Autodesk Inventor part; units mm, degrees
ref_plane "YZ Plane" through (0, 0, 0) normal (1, 0, 0) x (0, 1, 0)
ref_plane "XZ Plane" through (0, 0, 0) normal (0, 1, 0) x (-1, 0, 0)
ref_plane "XY Plane" through (0, 0, 0) normal (0, 0, 1) x (1, 0, 0)
sketch "Sketch1" plane through (0, 0, 0) normal (0, 0, 1) x (1, 0, 0)
  circle A0 centre (0, 0) radius 20.05
  dimension "d0" = 40.1
extrude "Extrusion1" add sketch "Sketch1" along normal blind 17.5
sketch "Sketch2" plane through (0, 0, 17.5) normal (0, 0, 1) x (1, 0, 0)
  line L0 (-16.51, 0) -> (-20.1782, -2.1178)
  line L1 (-20.1782, -2.1178) -> (-20.1782, 2.1178)
  line L2 (-20.1782, 2.1178) -> (-16.51, 0)
  line L3 (-16.1492, -3.4326) -> (-19.297, -6.2669)
  line L4 (-19.297, -6.2669) -> (-20.1776, -2.1237)
  line L5 (-20.1776, -2.1237) -> (-16.1492, -3.4326)
  line L6 (-15.0827, -6.7152) -> (-17.5723, -10.142)
  line L7 (-17.5723, -10.142) -> (-19.2951, -6.2725)
  line L8 (-19.2951, -6.2725) -> (-15.0827, -6.7152)
  line L9 (-13.3569, -9.7043) -> (-15.0797, -13.5738)
  line L10 (-15.0797, -13.5738) -> (-17.5694, -10.1471)
  line L11 (-17.5694, -10.1471) -> (-13.3569, -9.7043)
  line L12 (-11.0474, -12.2693) -> (-11.928, -16.4125)
  line L13 (-11.928, -16.4125) -> (-15.0757, -13.5782)
  line L14 (-15.0757, -13.5782) -> (-11.0474, -12.2693)
  line L15 (-8.255, -14.2981) -> (-8.255, -18.5338)
  line L16 (-8.255, -18.5338) -> (-11.9232, -16.4159)
  line L17 (-11.9232, -16.4159) -> (-8.255, -14.2981)
  line L18 (-5.1019, -15.702) -> (-4.2212, -19.8451)
  line L19 (-4.2212, -19.8451) -> (-8.2496, -18.5362)
  line L20 (-8.2496, -18.5362) -> (-5.1019, -15.702)
  line L21 (-1.7258, -16.4196) -> (-0.003, -20.2891)
  line L22 (-0.003, -20.2891) -> (-4.2154, -19.8463)
  line L23 (-4.2154, -19.8463) -> (-1.7258, -16.4196)
  line L24 (1.7258, -16.4196) -> (4.2154, -19.8463)
  line L25 (4.2154, -19.8463) -> (0.003, -20.2891)
  line L26 (0.003, -20.2891) -> (1.7258, -16.4196)
  line L27 (5.1019, -15.702) -> (8.2496, -18.5362)
  line L28 (8.2496, -18.5362) -> (4.2212, -19.8451)
  line L29 (4.2212, -19.8451) -> (5.1019, -15.702)
  line L30 (8.255, -14.2981) -> (11.9232, -16.4159)
  line L31 (11.9232, -16.4159) -> (8.255, -18.5338)
  line L32 (8.255, -18.5338) -> (8.255, -14.2981)
  line L33 (11.0474, -12.2693) -> (15.0757, -13.5782)
  line L34 (15.0757, -13.5782) -> (11.928, -16.4125)
  line L35 (11.928, -16.4125) -> (11.0474, -12.2693)
  line L36 (13.3569, -9.7043) -> (17.5694, -10.1471)
  line L37 (17.5694, -10.1471) -> (15.0797, -13.5738)
  line L38 (15.0797, -13.5738) -> (13.3569, -9.7043)
  line L39 (15.0827, -6.7152) -> (19.2951, -6.2725)
  line L40 (19.2951, -6.2725) -> (17.5723, -10.142)
  line L41 (17.5723, -10.142) -> (15.0827, -6.7152)
  line L42 (16.1492, -3.4326) -> (20.1776, -2.1237)
  line L43 (20.1776, -2.1237) -> (19.297, -6.2669)
  line L44 (19.297, -6.2669) -> (16.1492, -3.4326)
  line L45 (16.51, 0) -> (20.1782, 2.1178)
  line L46 (20.1782, 2.1178) -> (20.1782, -2.1178)
  line L47 (20.1782, -2.1178) -> (16.51, 0)
  line L48 (16.1492, 3.4326) -> (19.297, 6.2669)
  line L49 (19.297, 6.2669) -> (20.1776, 2.1237)
  line L50 (20.1776, 2.1237) -> (16.1492, 3.4326)
  line L51 (15.0827, 6.7152) -> (17.5723, 10.142)
  line L52 (17.5723, 10.142) -> (19.2951, 6.2725)
  line L53 (19.2951, 6.2725) -> (15.0827, 6.7152)
  line L54 (13.3569, 9.7043) -> (15.0797, 13.5738)
  line L55 (15.0797, 13.5738) -> (17.5694, 10.1471)
  line L56 (17.5694, 10.1471) -> (13.3569, 9.7043)
  line L57 (11.0474, 12.2693) -> (11.928, 16.4125)
  line L58 (11.928, 16.4125) -> (15.0757, 13.5782)
  line L59 (15.0757, 13.5782) -> (11.0474, 12.2693)
  line L60 (8.255, 14.2981) -> (8.255, 18.5338)
  line L61 (8.255, 18.5338) -> (11.9232, 16.4159)
  line L62 (11.9232, 16.4159) -> (8.255, 14.2981)
  line L63 (5.1019, 15.702) -> (4.2212, 19.8451)
  line L64 (4.2212, 19.8451) -> (8.2496, 18.5362)
  line L65 (8.2496, 18.5362) -> (5.1019, 15.702)
  line L66 (1.7258, 16.4196) -> (0.003, 20.2891)
  line L67 (0.003, 20.2891) -> (4.2154, 19.8463)
  line L68 (4.2154, 19.8463) -> (1.7258, 16.4196)
  line L69 (-1.7258, 16.4196) -> (-4.2154, 19.8463)
  line L70 (-4.2154, 19.8463) -> (-0.003, 20.2891)
  line L71 (-0.003, 20.2891) -> (-1.7258, 16.4196)
  line L72 (-5.1019, 15.702) -> (-8.2496, 18.5362)
  line L73 (-8.2496, 18.5362) -> (-4.2212, 19.8451)
  line L74 (-4.2212, 19.8451) -> (-5.1019, 15.702)
  line L75 (-8.255, 14.2981) -> (-11.9232, 16.4159)
  line L76 (-11.9232, 16.4159) -> (-8.255, 18.5338)
  line L77 (-8.255, 18.5338) -> (-8.255, 14.2981)
  line L78 (-11.0474, 12.2693) -> (-15.0757, 13.5782)
  line L79 (-15.0757, 13.5782) -> (-11.928, 16.4125)
  line L80 (-11.928, 16.4125) -> (-11.0474, 12.2693)
  line L81 (-13.3569, 9.7043) -> (-17.5694, 10.1471)
  line L82 (-17.5694, 10.1471) -> (-15.0797, 13.5738)
  line L83 (-15.0797, 13.5738) -> (-13.3569, 9.7043)
  line L84 (-15.0827, 6.7152) -> (-19.2951, 6.2725)
  line L85 (-19.2951, 6.2725) -> (-17.5723, 10.142)
  line L86 (-17.5723, 10.142) -> (-15.0827, 6.7152)
  line L87 (-16.1492, 3.4326) -> (-20.1776, 2.1237)
  line L88 (-20.1776, 2.1237) -> (-19.297, 6.2669)
  line L89 (-19.297, 6.2669) -> (-16.1492, 3.4326)
  point P0 (0, 0)
  point P1 (-18.9555, 0)
  point P2 (-18.5413, -3.9411)
  point P3 (-17.3167, -7.7099)
  point P4 (-15.3353, -11.1418)
  point P5 (-12.6837, -14.0867)
  point P6 (-9.4777, -16.4159)
  point P7 (-5.8576, -18.0277)
  point P8 (-1.9814, -18.8517)
  point P9 (1.9814, -18.8517)
  point P10 (5.8576, -18.0277)
  point P11 (9.4777, -16.4159)
  point P12 (12.6837, -14.0867)
  point P13 (15.3353, -11.1418)
  point P14 (17.3167, -7.7099)
  point P15 (18.5413, -3.9411)
  point P16 (18.9555, 0)
  point P17 (18.5413, 3.9411)
  point P18 (17.3167, 7.7099)
  point P19 (15.3353, 11.1418)
  point P20 (12.6837, 14.0867)
  point P21 (9.4777, 16.4159)
  point P22 (5.8576, 18.0277)
  point P23 (1.9814, 18.8517)
  point P24 (-1.9814, 18.8517)
  point P25 (-5.8576, 18.0277)
  point P26 (-9.4777, 16.4159)
  point P27 (-12.6837, 14.0867)
  point P28 (-15.3353, 11.1418)
  point P29 (-17.3167, 7.7099)
  point P30 (-18.5413, 3.9411)
  dimension "d5" = 360
extrude "Extrusion2" cut sketch "Sketch2" against normal through all
sketch "Sketch3" plane through (0, 0, 0) normal (0, 0, -1) x (-1, 0, 0)
  point P0 (0, 0)
  point P1 (0, 0)
hole "Hole1" at (0, 0, 0) at (0, 0, 0) direction (0, 0, 1) diameter 6 end through all
properties part number "gear(1.5 inch with 2mm extra)"
Could you check a few things on this model? Use its own coordinates, in mm. A direction names the side the tool comes from. Give positions to 0.01 mm unless a question says otherwise; leave off trailing zeros. Order: outer loops, then holes, each group sorted by start corner. A loop starts at its lowest first (then second) coordinate and runs counter-clockwise, first axis right, second up. Notation, with made-up numbers: (79.5, 62) -> (126.5, 62) arc R21 cw to (126.5, 91) -> close; hole circle Ø8 at (65, 7). An arc over 180 degrees is marked (long way). Return JSON: item names as keys, results as strings.
1. For pin 1 Ø1.2 at (y, z) = (15.5, 9.5) entering from -X; pin 2 Ø5 at (x, z) = (13, 14) entering from -Y; pin 3 Ø1 at (y, z) = (-2.5, 3) entering from +X; pin 4 Ø1 at (x, z) = (3.5, 3) entering from +Y, each with a flat end and sliding along its axis, tell me the tip position at first contact or that it passes through.
Answer list:
{"pin 1": "stops at x = -11.86", "pin 2": "stops at y = -16.28", "pin 3": "stops at x = 19.95", "pin 4": "stops at y = 19.55"}
2. Imagine slicing it at C-C on x = -9. List the corners of the cut face in (y, z) for me, then the cut area to 3 significant figures.
Answer list:
{"outline": "(-14.73, 0) -> (14.73, 0) -> (14.73, 17.5) -> (-14.73, 17.5) -> close", "area": "515 mm2"}
3. Imagine slicing it at B-B on y = 11. List the corners of the cut face in (x, z) for me.
Answer list:
{"outline": "(-13.93, 0) -> (13.93, 0) -> (13.93, 17.5) -> (-13.93, 17.5) -> close"}
4. Thinking about a two-plate mould opening in X: for faces 6 (the flat face through (18.01, -2.83, 8.87)), 7 (the flat face through (-18.1, -2.8, 8.9)), 8 (the flat face through (-6.6, -17.05, 8.87)), which applies, pulls with the +X half, pulls with the -X half, needs draft (parallel to the pull), parting line crosses it, or undercut?
Answer list:
{"face 6": "pulls with the +X half", "face 7": "pulls with the -X half", "face 8": "undercut"}
5. Imagine slicing it at A-A on x = 14. List the corners of the cut face in (y, z) for me.
Answer list:
{"outline": "(-13.23, 0) -> (-11.15, 0) -> (-11.15, 17.5) -> (-13.23, 17.5) -> close; (-9.77, 0) -> (9.77, 0) -> (9.77, 17.5) -> (-9.77, 17.5) -> close; (11.15, 0) -> (13.23, 0) -> (13.23, 17.5) -> (11.15, 17.5) -> close"}
6. I need wall thicknesses on line 1 (Y direction, x = 0, z = 4.75); line 2 (X direction, y = 18, z = 7) (3 decimals); line 3 (X direction, y = 14.5, z = 5.5) (3 decimals). Which ranges of each line are inside material? Lowest first, please. Write a range as from..to.
Answer list:
{"line 1": "y = -20.05..-3, 3..20.05", "line 2": "x = -8.255..-7.654, -4.613..-2.874, -1.022..1.022, 2.874..4.613, 7.654..8.255", "line 3": "x = -11.522..-8.605, -8.255..8.255, 8.605..11.522"}
7. On a 3-axis mill with a long thin cutter (end or side, diameter ignored), from which of +Z, -Z, +X, -X, +Y, -Y can I reach the whole of each face in a straight line? I mean faces 1 (the flat face through (-8.255, -16, 9)), 2 (the flat face through (-16.27, 8.35, 8.87)), 3 (the flat face through (16.27, -8.35, 8.87)), 4 (the flat face through (12.911, -12.875, 8.872)), 5 (the flat face through (-4.683, 17.673, 8.872)). Say none if no direction works.
Answer list:
{"face 1": "+Z, -Z, -Y", "face 2": "+Z, -Z, -X", "face 3": "+Z, -Z, +X", "face 4": "+Z, -Z", "face 5": "+Z, -Z, +Y"}
